```python
from build123d import *

# Parameters (mm, degrees)
BOSS_EXTRUDE1_DEPTH = 6.35
SKETCH2_R           = 2.286
CUT_EXTRUDE1_DEPTH  = 99.078502682
FILLET2_R           = 2.54


with BuildPart() as part:
    # Sketch1 → Boss-Extrude1 (new body)
    with BuildSketch(Plane.XY):
        Polygon((0, 0), (50.8, 0), (87.535311894, -43.779439924), (36.735311894, -43.779439924), align=None)
    extrude(amount=BOSS_EXTRUDE1_DEPTH)

    # Sketch2 → Cut-Extrude1 (cut, through all)
    with BuildSketch(Plane.XY.offset(6.35)):
        with Locations((74.835311894, -37.429439924)):
            Circle(SKETCH2_R)
        with Locations((49.435311894, -37.429439924)):
            Circle(SKETCH2_R)
    extrude(amount=-CUT_EXTRUDE1_DEPTH, mode=Mode.SUBTRACT)

    # Fillet1
    # an asymmetric fillet: 43.18, 35.56 mm, written as the material it takes off along each edge
    with BuildSketch(Plane(origin=(50.8, 0, -66.322759672), x_dir=(-1, 0, 0), z_dir=(0, 0, 1))) as fillet1_piece_1:
        with BuildLine():
            Bezier((26.529103869, 0), (0, 0), (-6.548695185, 7.804431014), weights=[1, 0.906307787, 1])
            Line((-6.548695185, 7.804431014), (0, 0))
            Line((0, 0), (26.529103869, 0))
        make_face()
    extrude(amount=138.995519344, mode=Mode.SUBTRACT)

    # Fillet2
    fillet2_edges = [part.edges().sort_by_distance(p)[0] for p in [
        (87.535311894, -43.779439924, 3.175),
        (0, 0, 3.175),
        (36.735311894, -43.779439924, 3.175),
    ]]
    fillet(fillet2_edges, radius=FILLET2_R)


solid = part.part
```
Check sheet for the modelled part. Datum: model origin and axes. Units: mm. Round coordinates to 2 decimals unless told otherwise and drop trailing zeros. Loops run counter-clockwise (first coordinate to the right, second up) from the corner with the lowest first, then second, coordinate; pieces in that order, holes last. Notation, with made-up numbers: (79.25, -10.75) -> (128.25, -10.75) arc R29 ccw to (128.25, 25.25) -> close; hole circle Ø7 at (4.5, -27.5). An arc over 180 degrees is marked (long way). Answer in a Markdown table with one row per item.
Q1. Go/stop test with flat-tipped pins: P1, Ø5, axis at x = 28, y = -38, coming from the -Z side; P2, Ø1, axis at y = -11.5, z = 5, coming from the +X side; P3, Ø1, axis at x = 13, z = 3.5, coming from the -Y side; P4, Ø3, axis at y = -16, z = 1, coming from the -X side. Record where each tip stops, or that it passes through.
Data:
| item | result |
|---|---|
| P1 | passes through |
| P2 | stops at x = 60.87 |
| P3 | stops at y = -16.09 |
| P4 | stops at x = 12.17 |
Q2. Sectioned sample at C-C on x = 67. Enter the section's corners in (y, z), then the cut area to 3 significant figures.
Data:
| item | result |
|---|---|
| outline | (-43.78, 0) -> (-19.31, 0) -> (-19.31, 6.35) -> (-43.78, 6.35) -> close |
| area | 155 mm^2 |
Q3. Release check for a two-part mould opening along Y. For faces 1 (the face through (70.5, -23.48, 3.13)), 2 (the face through (36.832, -43.535, 3.219)), 3 (the face through (51.6, -36.7, 3.2)) record: released by +Y, released by -Y, zero draft, split by the parting line, or undercut.
Data:
| item | result |
|---|---|
| face 1 | released by +Y |
| face 2 | released by -Y |
| face 3 | undercut |
Q4. Thickness scan on L1, parallel to X at y = -36.5, z = 0.5; L2, parallel to Y at x = 79.5, z = 3.25; L3, parallel to Y at x = 56, z = 3.75. Record the ranges inside material, lowest first.
Data:
| item | result |
|---|---|
| L1 | x = 30.63 to 47.35, 51.52 to 72.75, 76.92 to 81.43 |
| L2 | y = -43.78 to -34.2 |
| L3 | y = -43.78 to -6.49 |
Q5. Sectioned sample at A-A on y = -36.5. Enter the section's corners in (x, z), then the cut area to 3 significant figures.
Data:
| item | result |
|---|---|
| outline | (30.63, 0) -> (47.35, 0) -> (47.35, 6.35) -> (30.63, 6.35) -> close; (51.52, 0) -> (72.75, 0) -> (72.75, 6.35) -> (51.52, 6.35) -> close; (76.92, 0) -> (81.43, 0) -> (81.43, 6.35) -> (76.92, 6.35) -> close |
| area | 270 mm^2 |
Q6. Sectioned sample at D-D on y = -25.5. Enter the section's corners in (x, z).
Data:
| item | result |
|---|---|
| outline | (21.4, 0) -> (72.2, 0) -> (72.2, 6.35) -> (21.4, 6.35) -> close |
Q7. Sectioned sample at B-B on z = 5.25. Give the number of separate pieces and of enclosed holes in the cut face, then the cut area to 3 significant figures.
Data:
| item | result |
|---|---|
| separate pieces | 1 |
| enclosed holes | 2 |
| area | 2,140 mm^2 |
